```python
from build123d import *

# Parameters (mm, degrees)
BOSS_EXTRUDE1_DEPTH = 63.5
SKETCH2_OUTSIDE_W   = 21.185
SKETCH2_OUTSIDE_H   = 22.155
SKETCH2_OUTSIDE_R   = 1.143
CUT_EXTRUDE1_DEPTH  = 6.35
SKETCH3_OUTSIDE_W   = 21.185
SKETCH3_OUTSIDE_H   = 22.155
SKETCH3_OUTSIDE_R   = 3.048
CUT_EXTRUDE2_DEPTH  = 12.7
SKETCH4_OUTSIDE_W   = 21.185
SKETCH4_OUTSIDE_H   = 22.155
SKETCH4_OUTSIDE_R   = 2.54
CUT_EXTRUDE3_DEPTH  = 2.54


with BuildPart() as part:
    # Sketch1 → Boss-Extrude1 (new body)
    with BuildSketch(Plane(origin=(0, 0, 0), x_dir=(1, 0, 0), z_dir=(0, 1, 0))):
        Polygon((3.310191022, -4.420128359), (3.310191022, -0.762528359), (0.140765019, 1.063061018), (-3.028660983, -0.762528359), (-3.028660983, -4.420128359), (0.140765019, -6.245717737), align=None)
    extrude(amount=BOSS_EXTRUDE1_DEPTH)

    # Sketch2 outside → Cut-Extrude1 (cut)
    with BuildSketch(Plane(origin=(0, 63.5, 0), x_dir=(1, 0, 0), z_dir=(0, 1, 0))):
        with Locations((0.1405, -2.5915)):
            Rectangle(SKETCH2_OUTSIDE_W, SKETCH2_OUTSIDE_H)
        with Locations(Location((0.146339017, -2.591328359, 0), (0, 0, 270))):
            Circle(SKETCH2_OUTSIDE_R, mode=Mode.SUBTRACT)
    extrude(amount=-CUT_EXTRUDE1_DEPTH, mode=Mode.SUBTRACT)

    # Sketch3 outside → Cut-Extrude2 (cut)
    with BuildSketch(Plane.XZ):
        with Locations((0.1405, 2.5915)):
            Rectangle(SKETCH3_OUTSIDE_W, SKETCH3_OUTSIDE_H)
        with Locations(Location((0.152614949, 2.5845028, 0), (0, 0, 270))):
            Circle(SKETCH3_OUTSIDE_R, mode=Mode.SUBTRACT)
    extrude(amount=-CUT_EXTRUDE2_DEPTH, mode=Mode.SUBTRACT)

    # Sketch4 outside → Cut-Extrude3 (cut)
    with BuildSketch(Plane(origin=(0, 2.54, 0), x_dir=(-1, 0, 0), z_dir=(0, -1, 0))):
        with Locations((-0.1405, -2.5915)):
            Rectangle(SKETCH4_OUTSIDE_W, SKETCH4_OUTSIDE_H)
        with Locations(Location((-0.140765019, -2.591328359, 0), (0, 0, 90))):
            Circle(SKETCH4_OUTSIDE_R, mode=Mode.SUBTRACT)
    extrude(amount=-CUT_EXTRUDE3_DEPTH, mode=Mode.SUBTRACT)


solid = part.part
```
Read the model definition and answer for the solid it produces. Units are mm, in the model's axes. A direction names the side the tool comes from. Round coordinates to 2 decimals unless told otherwise and drop trailing zeros. Write each loop counter-clockwise with the first axis right and the second up, starting at its lowest first coordinate (ties: lowest second). Pieces come first, ordered by that corner, then holes. Notation, with made-up numbers: (16, -14.75) -> (49, -14.75) arc R22 ccw to (49, -6.75) -> close; hole circle Ø3 at (22, 87). An arc over 180 degrees is marked (long way). Answer in a Markdown table with one row per item. Add a question column.
1) Which of the six approach directions +Z, -Z, +X, -X, +Y, -Y give full straight-line access (tool end or side, diameter ignored) to faces 4 (the face through (-0.549, 60.369, 1.684)), 5 (the face through (2.66, 3.79, 2.92)), 6 (the face through (-1.015, 1.252, -0.231))?
2) Given P1, Ø1.5, axis at x = 2, y = 55, coming from the -Z side; P2, Ø3, axis at x = 2, y = 37.5, coming from the -Z side, each flat-ended and moving along its own axis, determine where each tip first touches the part or whether it passes through.
3) Find section D-D, the plane y = 10.5. Determine the outline of the cut face in (x, z).
4) Determine the mould class of faces 1 (the face through (-1.3, 57.15, 2.5)), 2 (the face through (3.31, 35, 3)), 3 (the face through (1, 5.08, 0)) for opening direction Y: pulls with the +Y half, pulls with the -Y half, needs draft (parallel to the pull), parting line crosses it, or undercut.
5) Find section C-C, the plane z = 3. Determine the outline of the cut face in (x, y), and give its area (3 significant figures).
6) Consider line 1 (Y direction, x = 2, z = 0.75); line 2 (Y direction, x = 1.25, z = 4.75); line 3 (Y direction, x = 3.25, z = 3.75). Determine where each line is inside the solid, lowest interval first.
7) Find section A-A, the plane x = -1.75. Determine the outline of the cut face in (y, z).
8) Find section B-B, the plane y = 33. Determine the outline of the cut face in (x, z).
Findings below:
| question | item | result |
|---|---|---|
| 1 | face 4 | +Y |
| 1 | face 5 | none |
| 1 | face 6 | -Y |
| 2 | P1 | z = -0.42 |
| 2 | P2 | z = -0.86 |
| 3 | outline | circle Ø6.1 at (0.15, 2.58) |
| 4 | face 1 | pulls with the +Y half |
| 4 | face 2 | needs draft |
| 4 | face 3 | undercut |
| 5 | outline | (-3.03, 12.7) -> (-2.87, 12.7) -> (-2.87, 5.08) -> (-2.37, 5.08) -> (-2.37, 2.54) -> (-2.87, 2.54) -> (-2.87, 0) -> (3.17, 0) -> (3.17, 2.54) -> (2.65, 2.54) -> (2.65, 5.08) -> (3.17, 5.08) -> (3.17, 12.7) -> (3.31, 12.7) -> (3.31, 57.15) -> (1.21, 57.15) -> (1.21, 63.5) -> (-0.92, 63.5) -> (-0.92, 57.15) -> (-3.03, 57.15) -> close |
| 5 | area | 369 mm² |
| 6 | line 1 | 0 to 2.54, 5.08 to 57.15 |
| 6 | line 2 | 0 to 57.15 |
| 6 | line 3 | 12.7 to 57.15 |
| 7 | outline | (0, 0.2) -> (2.54, 0.2) -> (2.54, 0.9) -> (5.08, 0.9) -> (5.08, 0.2) -> (12.7, 0.2) -> (12.7, 0.03) -> (57.15, 0.03) -> (57.15, 5.16) -> (12.7, 5.16) -> (12.7, 4.97) -> (5.08, 4.97) -> (5.08, 4.29) -> (2.54, 4.29) -> (2.54, 4.97) -> (0, 4.97) -> close |
| 8 | outline | (-3.03, 0.76) -> (0.14, -1.06) -> (3.31, 0.76) -> (3.31, 4.42) -> (0.14, 6.25) -> (-3.03, 4.42) -> close |
